Read the model definition and answer for the solid it produces. Units are mm, in the model's axes. Coordinates: 2 decimals unless noted, no trailing zeros. Write each loop counter-clockwise with the first axis right and the second up, starting at its lowest first coordinate (ties: lowest second). Pieces come first, ordered by that corner, then holes. Notation, with made-up numbers: M 48.5,-27.5 L 100.5,-27.5 A26 cw 100.5,-6.5 Z; hole C 23.25,0.5 d9. An arc over 180 degrees is marked long. Write item = value, one per line.
from build123d import *

# Parameters (mm, degrees)
SKETCH1_W                           = 325
SKETCH1_H                           = 190
PLATFORM_DEPTH                      = 3.175
SKETCH2_W                           = 112
SKETCH2_H                           = 75
MICROPLATE_CUTOUT_DEPTH             = 4.175
SKETCH3_R                           = 1
LEAD_NUT_HOLE_POSITIONS_DEPTH       = 4.175
SKETCH4_R                           = 2.125
LINEAR_BEARING_MOUNTING_HOLES_DEPTH = 4.175
LPATTERN1_COUNT                     = 2
LPATTERN1_PITCH                     = 138
SKETCH10_W                          = 152.5
SKETCH10_H                          = 12
CUT_EXTRUDE1_DEPTH                  = 4.175
CHAMFER1_SIZE                       = 27
CHAMFER1_SIZE2                      = 138.902958431
FILLET1_R                           = 5
M3X0_5_TAPPED_HOLE1_D               = 2.5
M5X0_8_TAPPED_HOLE1_D               = 4.2
CUT_EXTRUDE3_DEPTH                  = 4.175
FILLET3_R                           = 3


with BuildPart() as part:
    # Sketch1 → Platform (new body)
    with BuildSketch(Plane(origin=(0, 0, 0), x_dir=(1, 0, 0), z_dir=(0, 1, 0))):
        Rectangle(SKETCH1_W, SKETCH1_H)
    extrude(amount=PLATFORM_DEPTH)

    # Sketch2 → Microplate Cutout (cut, through all)
    with BuildSketch(Plane(origin=(0, 3.175, 0), x_dir=(1, 0, 0), z_dir=(0, 1, 0))):
        with Locations((-94, 0)):
            Rectangle(SKETCH2_W, SKETCH2_H)
    extrude(amount=-MICROPLATE_CUTOUT_DEPTH, mode=Mode.SUBTRACT)

    # Sketch3 → Lead Nut Hole Positions (cut, through all)
    with BuildSketch(Plane(origin=(0, 3.175, 0), x_dir=(1, 0, 0), z_dir=(0, 1, 0))):
        with Locations((140.5, 20)):
            Circle(SKETCH3_R)
        with Locations((154.5, 20)):
            Circle(SKETCH3_R)
        with Locations((154.5, -20)):
            Circle(SKETCH3_R)
        with Locations((140.5, -20)):
            Circle(SKETCH3_R)
    extrude(amount=-LEAD_NUT_HOLE_POSITIONS_DEPTH, mode=Mode.SUBTRACT)

    # Sketch4 → Linear Bearing Mounting Holes (cut, through all)
    with BuildSketch(Plane(origin=(0, 3.175, 0), x_dir=(1, 0, 0), z_dir=(0, 1, 0))):
        with Locations((17.5, 88)):
            Circle(SKETCH4_R)
        with Locations((17.5, 64)):
            Circle(SKETCH4_R)
        with Locations((-0.5, 88)):
            Circle(SKETCH4_R)
        with Locations((-0.5, 64)):
            Circle(SKETCH4_R)
        with Locations((-0.5, -64)):
            Circle(SKETCH4_R)
        with Locations((-0.5, -88)):
            Circle(SKETCH4_R)
        with Locations((17.5, -64)):
            Circle(SKETCH4_R)
        with Locations((17.5, -88)):
            Circle(SKETCH4_R)
    linear_bearing_mounting_holes = extrude(amount=-LINEAR_BEARING_MOUNTING_HOLES_DEPTH, mode=Mode.SUBTRACT)

    # LPattern1: Linear Bearing Mounting Holes ×2
    with Locations(*[(i * LPATTERN1_PITCH, 0, 0) for i in range(1, LPATTERN1_COUNT)]):
        add(linear_bearing_mounting_holes, mode=Mode.SUBTRACT)

    # Sketch10 → Cut-Extrude1 (cut, through all)
    with BuildSketch(Plane(origin=(0, 3.175, 0), x_dir=(1, 0, 0), z_dir=(0, 1, 0))):
        with Locations((-86.25, 89)):
            Rectangle(SKETCH10_W, SKETCH10_H)
        with Locations((-86.25, -89)):
            Rectangle(SKETCH10_W, SKETCH10_H)
    extrude(amount=-CUT_EXTRUDE1_DEPTH, mode=Mode.SUBTRACT)

    # Chamfer1
    chamfer1_edges = [part.edges().sort_by_distance(p)[0] for p in [
        (-162.5, 1.5875, -83),
        (-162.5, 1.5875, 83),
    ]]
    chamfer1_side = [part.faces().sort_by_distance(p)[0] for p in [
        (-162.5, 1.5875, 0),
    ]]
    chamfer(chamfer1_edges, length=CHAMFER1_SIZE, length2=CHAMFER1_SIZE2, reference=chamfer1_side[0])

    # Fillet1
    fillet1_edges = [part.edges().sort_by_distance(p)[0] for p in [
        (-10, 1.5875, -95),
        (-10, 1.5875, -83),
        (-10, 1.5875, 83),
        (-10, 1.5875, 95),
        (-23.597041569, 1.5875, -83),
        (-162.5, 1.5875, 56),
        (-162.5, 1.5875, -56),
        (-23.597041569, 1.5875, 83),
        (-38, 1.5875, -37.5),
        (-38, 1.5875, 37.5),
        (-150, 1.5875, 37.5),
        (-150, 1.5875, -37.5),
        (162.5, 1.5875, 95),
        (162.5, 1.5875, -95),
    ]]
    fillet(fillet1_edges, radius=FILLET1_R)

    # M3x0.5 Tapped Hole1 (through all)
    with Locations(Plane(origin=(0, 3.175, 0), x_dir=(1, 0, 0), z_dir=(0, 1, 0))):
        with Locations((-94, 0), (-34, 49), (-154, -49), (-154, 49), (-34, -49)):
            Hole(M3X0_5_TAPPED_HOLE1_D / 2)

    # M5x0.8 Tapped Hole1 (through all)
    with Locations(Plane(origin=(0, 3.175, 0), x_dir=(1, 0, 0), z_dir=(0, 1, 0))):
        with Locations((154.5, 20), (140.5, 20), (154.5, -20), (140.5, -20)):
            Hole(M5X0_8_TAPPED_HOLE1_D / 2)

    # Sketch12 → Cut-Extrude3 (cut, through all)
    with BuildSketch(Plane(origin=(0, 3.175, 0), x_dir=(1, 0, 0), z_dir=(0, 1, 0))):
        Polygon((122.5, 22.461125504), (31.5, 75), (122.5, 75), align=None)
        Polygon((122.5, 10), (31.5, 62.538874496), (31.5, 10), align=None)
        Polygon((31.5, -10), (122.5, -10), (31.5, -62.538874496), align=None)
        Polygon((31.5, -75), (122.5, -75), (122.5, -22.461125504), align=None)
    extrude(amount=-CUT_EXTRUDE3_DEPTH, mode=Mode.SUBTRACT)

    # Fillet3
    fillet3_edges = [part.edges().sort_by_distance(p)[0] for p in [
        (122.5, 1.5875, -10),
        (31.5, 1.5875, -10),
        (31.5, 1.5875, -62.538874496),
        (122.5, 1.5875, 22.461125504),
        (122.5, 1.5875, 75),
        (31.5, 1.5875, 75),
        (31.5, 1.5875, 62.538874496),
        (31.5, 1.5875, 10),
        (122.5, 1.5875, 10),
        (122.5, 1.5875, -75),
        (122.5, 1.5875, -22.461125504),
        (31.5, 1.5875, -75),
    ]]
    fillet(fillet3_edges, radius=FILLET3_R)


solid = part.part
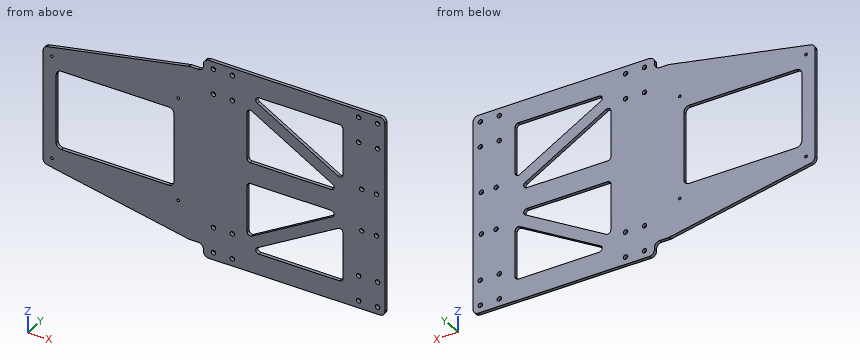
Item 1: Consider line 1 along Z through (x, y) = (137.5, 1.2) (3 decimals); line 2 along Z through (x, y) = (-33, 0.8); line 3 along X through (y, z) = (1.05, -44). Determine where each line is inside the solid, lowest interval first. Write a range as from..to.
Worked answers:
line_1 = -95..-90.125, -85.875..-66.125, -61.875..61.875, 66.125..85.875, 90.125..95
line_2 = -81.17..-49.75, -48.25..48.25, 49.75..81.17
line_3 = -162.5..31.5, 63.61..85.19, 122.5..162.5
Item 2: Find section D-D (x = -104). Determine the outline of the cut face in (y, z) (3 decimals), and give its area (3 significant figures).
Worked answers:
outline = M 0,-67.371 L 3.175,-67.371 L 3.175,-37.5 L 0,-37.5 Z; M 0,37.5 L 3.175,37.5 L 3.175,67.371 L 0,67.371 Z
area = 190 mm²
Item 3: Find section A-A (x = -63.5). Determine the outline of the cut face in (y, z) (3 decimals), and give its area (3 significant figures).
Worked answers:
outline = M 0,-75.244 L 3.175,-75.244 L 3.175,-37.5 L 0,-37.5 Z; M 0,37.5 L 3.175,37.5 L 3.175,75.244 L 0,75.244 Z
area = 240 mm²
Item 4: Find section C-C (x = 56). Determine the outline of the cut face in (y, z) (3 decimals), and give its area (3 significant figures).
Worked answers:
outline = M 0,-95 L 3.175,-95 L 3.175,-75 L 0,-75 Z; M 0,-60.855 L 3.175,-60.855 L 3.175,-48.394 L 0,-48.394 Z; M 0,-10 L 3.175,-10 L 3.175,10 L 0,10 Z; M 0,48.394 L 3.175,48.394 L 3.175,60.855 L 0,60.855 Z; M 0,75 L 3.175,75 L 3.175,95 L 0,95 Z
area = 270 mm²
Item 5: Flat-ended cylindrical pins translate along their axes: pin 1 (1 mm diameter, centred on x = -20, y = 1, fed in from -Z); pin 2 (1 mm diameter, centred on x = -115, y = 1, fed in from +Z); pin 3 (1.6 mm diameter, centred on x = -18, y = 1.5, fed in from +Z). Find the tip coordinate at first contact, or state that the pin passes through.
Worked answers:
pin_1 = -83
pin_2 = 65.33
pin_3 = 83
Item 6: Find section B-B (y = 0.9). State how many separate pieces and enclosed holes the cut face has, and give its area (3 significant figures).
Worked answers:
separate_pieces = 1
enclosed_holes = 29
area = 36,200 mm²
